from build123d import *

# Parameters (mm, degrees)
SKETCH1_W                                    = 50.8
SKETCH1_H                                    = 25.4
BOSS_EXTRUDE1_DEPTH                          = 12.7
CBORE_FOR_10_SOCKET_HEAD_CAP_SCREW1_AT_COUNT = 2
CBORE_FOR_10_SOCKET_HEAD_CAP_SCREW1_AT_PITCH = 31.75
CBORE_FOR_10_SOCKET_HEAD_CAP_SCREW1_2_COUNT  = 2
CBORE_FOR_10_SOCKET_HEAD_CAP_SCREW1_2_PITCH  = 34.195796525
CBORE_FOR_10_SOCKET_HEAD_CAP_SCREW1_3_COUNT  = 2
CBORE_FOR_10_SOCKET_HEAD_CAP_SCREW1_3_PITCH  = 12.7
CUT_EXTRUDE1_REACH                           = 33.109
CUT_EXTRUDE2_DEPTH                           = 6.35
FILLET1_R                                    = 3.175


with BuildPart() as part:
    # Sketch1 → Boss-Extrude1 (new body)
    with BuildSketch(Plane.XY):
        Rectangle(SKETCH1_W, SKETCH1_H)
    extrude(amount=-BOSS_EXTRUDE1_DEPTH)

    # Sketch2 → CBORE for #10 Socket Head Cap Screw1 (revolve, cut)
    with BuildSketch(Plane(origin=(-15.875, 6.35, 0), x_dir=(0, -1, 0), z_dir=(1, 0, 0))):
        Polygon((0, 0), (0, 12.7), (2.5527, 12.7), (2.5527, 5.08), (4.7625, 5.08), (4.7625, 0.635), (5.3975, 0), align=None)
    cbore_for_10_socket_head_cap_screw1 = revolve(axis=Axis((-15.875, 6.35, 6.35), (0, 0, -1)), mode=Mode.SUBTRACT)

    # CBORE for #10 Socket Head Cap Screw1 at: CBORE for #10 Socket Head Cap Screw1 ×2
    with Locations(*[(i * CBORE_FOR_10_SOCKET_HEAD_CAP_SCREW1_AT_PITCH, 0, 0) for i in range(1, CBORE_FOR_10_SOCKET_HEAD_CAP_SCREW1_AT_COUNT)]):
        add(cbore_for_10_socket_head_cap_screw1, mode=Mode.SUBTRACT)

    # CBORE for _10 Socket Head Cap Screw1 2: CBORE for #10 Socket Head Cap Screw1 ×2
    with Locations(*[Vector(0.9284766908852594, -0.37139067635410367, 0) * (i * CBORE_FOR_10_SOCKET_HEAD_CAP_SCREW1_2_PITCH) for i in range(1, CBORE_FOR_10_SOCKET_HEAD_CAP_SCREW1_2_COUNT)]):
        add(cbore_for_10_socket_head_cap_screw1, mode=Mode.SUBTRACT)

    # CBORE for _10 Socket Head Cap Screw1 3: CBORE for #10 Socket Head Cap Screw1 ×2
    with Locations(*[(0, -i * CBORE_FOR_10_SOCKET_HEAD_CAP_SCREW1_3_PITCH, 0) for i in range(1, CBORE_FOR_10_SOCKET_HEAD_CAP_SCREW1_3_COUNT)]):
        add(cbore_for_10_socket_head_cap_screw1, mode=Mode.SUBTRACT)

    # Sketch4 → Cut-Extrude1 (cut, up to next)
    with BuildSketch(Plane.XY, mode=Mode.PRIVATE) as cut_extrude1_sk1:
        with BuildLine():
            Line((-6.35, 0), (-6.35, -12.7))
            Line((-6.35, -12.7), (6.35, -12.7))
            Line((6.35, -12.7), (6.35, 0))
            ThreePointArc((6.35, 0), (0, 6.35), (-6.35, 0))
        make_face()
    cut_extrude1_tool1 = extrude(cut_extrude1_sk1.sketch, amount=-CUT_EXTRUDE1_REACH, mode=Mode.PRIVATE) & part.part
    add(cut_extrude1_tool1.solids().sort_by_distance((0, -3.799576, 0))[0], mode=Mode.SUBTRACT)

    # Sketch5 → Cut-Extrude2 (cut)
    with BuildSketch(Plane(origin=(0, 0, -12.7), x_dir=(-1, 0, 0), z_dir=(0, 0, -1))):
        with BuildLine():
            Line((-11.1125, 0), (-11.1125, -12.7))
            Line((-11.1125, -12.7), (11.1125, -12.7))
            Line((11.1125, -12.7), (11.1125, 0))
            ThreePointArc((11.1125, 0), (0, 11.1125), (-11.1125, 0))
        make_face()
    extrude(amount=-CUT_EXTRUDE2_DEPTH, mode=Mode.SUBTRACT)

    # Fillet1
    # the kernel refuses this fillet: 3.175 mm, written as the material it takes off along each edge
    with BuildSketch(Plane(origin=(-22.225, 9.525, -3.175), x_dir=(-1, 0, 0), z_dir=(0, 1, 0))) as fillet1_piece_1_section:
        Polygon((0, 0), (FILLET1_R, 0), (FILLET1_R, FILLET1_R), (0, FILLET1_R), align=None)
    fillet1_piece_1 = extrude(amount=FILLET1_R, mode=Mode.PRIVATE)
    fillet1_piece_1 = fillet1_piece_1 - Plane(origin=(-22.225, 9.525, -3.175), x_dir=(0.7071067811865475, 0, -0.7071067811865475), z_dir=(0, 1, 0)) * Sphere(FILLET1_R, mode=Mode.PRIVATE)
    add(fillet1_piece_1, mode=Mode.SUBTRACT)
    with BuildSketch(Plane(origin=(22.225, 9.525, -3.175), x_dir=(1, 0, 0), z_dir=(0, 1, 0))) as fillet1_piece_2_section:
        Polygon((0, 0), (FILLET1_R, 0), (FILLET1_R, -FILLET1_R), (0, -FILLET1_R), align=None)
    fillet1_piece_2 = extrude(amount=FILLET1_R, mode=Mode.PRIVATE)
    fillet1_piece_2 = fillet1_piece_2 - Plane(origin=(22.225, 9.525, -3.175), x_dir=(-0.7071067811865475, 0, -0.7071067811865475), z_dir=(0, 1, 0)) * Sphere(FILLET1_R, mode=Mode.PRIVATE)
    add(fillet1_piece_2, mode=Mode.SUBTRACT)
    with BuildSketch(Plane(origin=(-25.4, -20.6375, 0), x_dir=(0, 0, -1), z_dir=(0, 1, 0)), Plane(origin=(25.4, 9.525, 0), x_dir=(0, 0, -1), z_dir=(0, -1, 0))) as fillet1_piece_3:
        with BuildLine():
            CenterArc((FILLET1_R, -FILLET1_R), FILLET1_R, 90, 90)
            Line((0, -FILLET1_R), (0, 0))
            Line((0, 0), (FILLET1_R, 0))
        make_face()
    extrude(amount=30.1625, mode=Mode.SUBTRACT)
    with BuildSketch(Plane(origin=(-22.225, 12.7, 0), x_dir=(0, 0, -1), z_dir=(1, 0, 0))) as fillet1_piece_4:
        with BuildLine():
            CenterArc((FILLET1_R, -FILLET1_R), FILLET1_R, 90, 90)
            Line((0, -FILLET1_R), (0, 0))
            Line((0, 0), (FILLET1_R, 0))
        make_face()
    extrude(amount=44.45, mode=Mode.SUBTRACT)
    with BuildSketch(Plane(origin=(-25.4, 12.7, -3.175), x_dir=(1, 0, 0), z_dir=(0, 0, -1))) as fillet1_piece_5:
        with BuildLine():
            CenterArc((FILLET1_R, FILLET1_R), FILLET1_R, 180, 90)
            Line((0, FILLET1_R), (0, 0))
            Line((0, 0), (FILLET1_R, 0))
        make_face()
    extrude(amount=17.4625, mode=Mode.SUBTRACT)
    with BuildSketch(Plane(origin=(25.4, 12.7, -3.175), x_dir=(-1, 0, 0), z_dir=(0, 0, -1))) as fillet1_piece_6:
        with BuildLine():
            CenterArc((FILLET1_R, -FILLET1_R), FILLET1_R, 90, 90)
            Line((0, -FILLET1_R), (0, 0))
            Line((0, 0), (FILLET1_R, 0))
        make_face()
    extrude(amount=17.4625, mode=Mode.SUBTRACT)


solid = part.part
Geometry: final body of the model. Coordinates: model frame, mm. A direction names the side the tool comes from. Round coordinates to 2 decimals unless told otherwise and drop trailing zeros. One line per question, with ' | ' between items.
(1) Pull-direction query (X, two-part tool) for faces 6 (the flat face through (-5, 5, -6.35)), 7 (the flat face through (-16, -12.7, -6)), 8 (the cylindrical face through (24.49, -1.43, -0.95)); classes: +X half, -X half, draft (parallel to the pull), parting line (faces both ways), or undercut.
Check result:
face 6: undercut | face 7: draft | face 8: +X half
(2) Contact query for flat-ended pins moving along their axis: P1, Ø4, axis at x = -8.5, y = -4, coming from the -Z side; P2, Ø5, axis at x = 18, y = -8, coming from the +Z side; P3, Ø2, axis at y = -6, z = -1.5, coming from the -X side. Output: stop coordinate, or through.
Check result:
P1: stops at z = -6.35 | P2: stops at z = -0.21 | P3: stops at x = -25.33
(3) Access query for faces 1 (the cylindrical face through (24.45, 11.79, -7.87)), 2 (the cylindrical face through (-0.24, 11.11, -9.57)), 3 (the flat face through (16, -12.7, -6)), 4 (the flat face through (-6.35, -6, -3)), 5 (the cylindrical face through (11.86, -8.91, -2.83)). Directions: +Z, -Z, +X, -X, +Y, -Y. A direction counts if a zero-diameter tool reaches every point of the face in a straight line with its end or side. Return the directions, or none.
Check result:
face 1: +Z, -Z, +X, +Y | face 2: -Z, -Y | face 3: +Z, -Z, +X, -X, -Y | face 4: +Z, -Z, -Y | face 5: +Z
(4) Material intervals for line 1 along X through (y, z) = (-6.35, -7.25); line 2 along X through (y, z) = (-6.35, -2.95); line 3 along X through (y, z) = (-0.75, -7.25), sorted ascending. Write a range as from..to.
Check result:
line 1: x = -25.4..-18.43, -13.32..-11.11, 11.11..13.32, 18.43..25.4 | line 2: x = -25.39..-20.64, -11.11..-6.35, 6.35..11.11, 20.64..25.39 | line 3: x = -25.4..-11.11, 11.11..25.4
(5) Cut plane A-A on y = -6.35. Give the number of separate pieces and of enclosed holes in the cut face, plus the area to 3 significant figures.
Check result:
separate pieces: 4 | enclosed holes: 0 | area: 244 mm2
